from build123d import *

# Parameters (mm, degrees)
PAD_DEPTH       = 6
SKETCH002_R     = 1.1
POCKET_DEPTH    = 6.001
POCKET001_DEPTH = 1.7
POCKET002_DEPTH = 1.7


with BuildPart() as part:
    # Sketch → Pad (new body)
    with BuildSketch(Plane.XY):
        with BuildLine():
            Line((0, 3), (13, 3))
            ThreePointArc((13, -3), (15.999986, 0), (13, 3))
            Line((0, -3), (13, -3))
            ThreePointArc((0, 3), (-3, 0), (0, -3))
        make_face()
    extrude(amount=PAD_DEPTH)

    # Sketch002 → Pocket (cut, through all)
    with BuildSketch(Plane.XY.offset(6)):
        Circle(SKETCH002_R)
        with Locations((13, 0)):
            Circle(SKETCH002_R)
    extrude(amount=-POCKET_DEPTH, mode=Mode.SUBTRACT)

    # Sketch003 → Pocket001 (cut)
    with BuildSketch(Plane.XY.offset(6)):
        Polygon((2.6, 0), (0.100002, -4.330128), (-3.899998, -4.330128), (-3.899998, 4.330126), (0.099998, 4.330126), align=None)
    extrude(amount=-POCKET001_DEPTH, mode=Mode.SUBTRACT)

    # Sketch004 → Pocket002 (cut)
    with BuildSketch(Plane(origin=(0, 0, 0), x_dir=(1, 0, 0), z_dir=(0, 0, -1))):
        Polygon((10.4, 0), (12.678902, 3.947175), (16.678902, 3.947175), (16.678902, -3.947175), (12.678903, -3.947175), align=None)
    extrude(amount=-POCKET002_DEPTH, mode=Mode.SUBTRACT)


solid = part.part
Geometry: final body of the model. Coordinates: model frame, mm. A direction names the side the tool comes from. Give positions to 0.01 mm unless a question says otherwise; leave off trailing zeros. Write each loop counter-clockwise with the first axis right and the second up, starting at its lowest first coordinate (ties: lowest second). Pieces come first, ordered by that corner, then holes. Notation, with made-up numbers: (49, 1) -> (72, 1) arc R17 ccw to (72, 25) -> close; hole circle Ø10 at (49.5, 85). An arc over 180 degrees is marked (long way). Answer in a Markdown table with one row per item.
(1) Pin query (flat end, axial travel): pin 1 (1.7 mm diameter, centred on x = 13.5, y = -1.5, fed in from -Z); pin 2 (1 mm diameter, centred on x = 14, z = 5, fed in from +Y); pin 3 (1 mm diameter, centred on y = 1, z = 2.5, fed in from -X). Return the tip coordinate at first contact, or that it passes through.
Answers below:
| item | result |
|---|---|
| pin 1 | z = 1.7 |
| pin 2 | y = 2.96 |
| pin 3 | x = -2.96 |
(2) Section query A-A on z = 2.4. Return loops of the section in (x, y).
Answers below:
| item | result |
|---|---|
| outline | (0, -3) -> (13, -3) arc R3 ccw to (13, 3) -> (0, 3) arc R3 ccw to start; hole circle Ø2.2 at (0, 0); hole circle Ø2.2 at (13, 0) |
(3) Set-up query: faces 1 (the flat face through (5, 0, 0)), 2 (the flat face through (11.278, 1.521, 0.838)), 3 (the flat face through (-1.4, 0, 4.3)). Return all of +Z, -Z, +X, -X, +Y, -Y with unobstructed straight access to the full face (end or side cutting, diameter ignored); none if empty.
Answers below:
| item | result |
|---|---|
| face 1 | -Z, +X, -X, +Y, -Y |
| face 2 | -Z, +X |
| face 3 | +Z, -X |
(4) Draft query along Y for faces 4 (the flat face through (11.254, -1.479, 0.838)), 5 (the cylindrical face through (-3, 0, 2)), 6 (the flat face through (9, 0, 6)). Return one class per face: +Y half, -Y half, draft (parallel to the pull), parting line (faces both ways), or undercut.
Answers below:
| item | result |
|---|---|
| face 4 | undercut |
| face 5 | parting line |
| face 6 | draft |
(5) Section query C-C on z = 4.9. Return loops of the section in (x, y), then the cut area to 3 significant figures.
Answers below:
| item | result |
|---|---|
| outline | (0.87, -3) -> (13, -3) arc R3 ccw to (13, 3) -> (0.87, 3) -> (2.6, 0) -> close; hole circle Ø2.2 at (13, 0) |
| area | 77.9 mm^2 |
(6) Section query D-D on y = -2.5. Return loops of the section in (x, z).
Answers below:
| item | result |
|---|---|
| outline | (-1.66, 0) -> (11.84, 0) -> (11.84, 1.7) -> (14.66, 1.7) -> (14.66, 6) -> (1.16, 6) -> (1.16, 4.3) -> (-1.66, 4.3) -> close |
(7) Section query B-B on y = 1.5. Return loops of the section in (x, z).
Answers below:
| item | result |
|---|---|
| outline | (-2.6, 0) -> (11.27, 0) -> (11.27, 1.7) -> (15.6, 1.7) -> (15.6, 6) -> (1.73, 6) -> (1.73, 4.3) -> (-2.6, 4.3) -> close |
(8) Ray query, line 1 along Y through (x, z) = (13, 4.8); line 2 along X through (y, z) = (0.75, 4.2); line 3 along X through (y, z) = (1, 2.25). Return the intervals inside material, ascending. Write a range as [from, to].
Answers below:
| item | result |
|---|---|
| line 1 | [-3, -1.1], [1.1, 3] |
| line 2 | [-2.9, -0.8], [0.8, 12.2], [13.8, 15.9] |
| line 3 | [-2.83, -0.46], [0.46, 12.54], [13.46, 15.83] |
